```python
from build123d import *

# Parameters (mm, degrees)
BOSS_EXTRUDE1_DEPTH            = 101.6
CUT_EXTRUDE2_REACH             = 142.769
SKETCH2_R                      = 2.9845
CUT_EXTRUDE2_DIRECTION_2_DEPTH = 141.768746531
SKETCH8_W                      = 3.81
SKETCH8_H                      = 101.6
BOSS_EXTRUDE3_DEPTH            = 101.6
CUT_EXTRUDE5_DEPTH             = 4.572
SKETCH24_W                     = 38.1
SKETCH24_H                     = 35.56
BOSS_EXTRUDE8_DEPTH            = 7.62
BOSS_EXTRUDE8_TAPER            = 20
SKETCH29_W                     = 5.08
SKETCH29_H                     = 16.309015266
BOSS_EXTRUDE10_DEPTH           = 21.59
CUT_EXTRUDE8_DEPTH             = 199.322792527
CUT_EXTRUDE8_DEPTH_BACK        = 199.322792527
SKETCH30_R                     = 2.54
FILLET8_R                      = 2.38
CUT_EXTRUDE9_DEPTH             = 3.81
FILLET9_R                      = 2.54


with BuildPart() as part:
    # Sketch1 → Boss-Extrude1 (new body)
    with BuildSketch(Plane.XY):
        Polygon((0, 0), (0, 76.2), (60.71935441, 76.2), (60.71935441, 69.85), (6.35, 69.85), (6.35, 8.89), (60.71935441, 8.89), (60.71935441, 0), align=None)
    extrude(amount=BOSS_EXTRUDE1_DEPTH)

    # Sketch2 → Cut-Extrude2 (cut, up to next)
    with BuildSketch(Plane(origin=(0, 0, 0), x_dir=(1, 0, 0), z_dir=(0, 1, 0)), mode=Mode.PRIVATE) as cut_extrude2_sk1:
        with Locations(Location((30.359677205, -50.8, 0), (0, 0, 270))):
            Circle(SKETCH2_R)
    cut_extrude2_tool1 = extrude(cut_extrude2_sk1.sketch, amount=CUT_EXTRUDE2_REACH, mode=Mode.PRIVATE) & part.part
    add(cut_extrude2_tool1.solids().sort_by_distance((30.359677, 0, 50.8))[0], mode=Mode.SUBTRACT)

    # Sketch2 → Cut-Extrude2 direction 2 (cut)
    with BuildSketch(Plane(origin=(0, 0, 0), x_dir=(1, 0, 0), z_dir=(0, 1, 0))):
        with Locations(Location((30.359677205, -50.8, 0), (0, 0, 270))):
            Circle(SKETCH2_R)
    extrude(amount=-CUT_EXTRUDE2_DIRECTION_2_DEPTH, mode=Mode.SUBTRACT)

    # Sketch8 → Boss-Extrude3 (add)
    with BuildSketch(Plane(origin=(0, 76.2, 0), x_dir=(1, 0, 0), z_dir=(0, 1, 0))):
        with Locations((1.905, -50.8)):
            Rectangle(SKETCH8_W, SKETCH8_H)
    extrude(amount=BOSS_EXTRUDE3_DEPTH)

    # Sketch20 → Cut-Extrude5 (cut)
    with BuildSketch(Plane(origin=(0, 8.89, 0), x_dir=(1, 0, 0), z_dir=(0, 1, 0))):
        Polygon((35.462369538, -53.693279158), (35.416676623, -47.827578391), (30.31398429, -44.934299233), (25.256984872, -47.906720842), (25.302677788, -53.772421609), (30.405370121, -56.665700767), align=None)
    extrude(amount=-CUT_EXTRUDE5_DEPTH, mode=Mode.SUBTRACT)

    # Sketch24 → Boss-Extrude8 (add)
    with BuildSketch(Plane(origin=(3.81, 0, 0), x_dir=(0, 0, -1), z_dir=(1, 0, 0))):
        with Locations((-50.8, 160.02)):
            Rectangle(SKETCH24_W, SKETCH24_H)
    extrude(amount=BOSS_EXTRUDE8_DEPTH, taper=BOSS_EXTRUDE8_TAPER)

    # Sketch29 → Boss-Extrude10 (add)
    with BuildSketch(Plane(origin=(11.43, 0, 0), x_dir=(0, 0, -1), z_dir=(1, 0, 0))):
        with Locations((-60.96, 160.02)):
            Rectangle(SKETCH29_W, SKETCH29_H)
        with Locations((-50.8, 160.02)):
            Rectangle(SKETCH29_W, SKETCH29_H)
        with Locations((-40.64, 160.02)):
            Rectangle(SKETCH29_W, SKETCH29_H)
    extrude(amount=BOSS_EXTRUDE10_DEPTH)

    # Sketch30 → Cut-Extrude8 (cut, two sides: drawn at the far end of the back side and taken through both)
    with BuildSketch(Plane.XY.offset(63.5).offset(-CUT_EXTRUDE8_DEPTH_BACK)):
        with Locations(Location((22.225, 163.094507633, 0), (0, 0, 180))):
            Circle(SKETCH30_R)
    extrude(amount=CUT_EXTRUDE8_DEPTH + CUT_EXTRUDE8_DEPTH_BACK, mode=Mode.SUBTRACT)

    # Fillet8
    fillet8_edges = [part.edges().sort_by_distance(p)[0] for p in [
        (33.02, 168.174507633, 40.64),
        (11.43, 160.02, 43.18),
        (11.43, 151.865492367, 40.64),
        (33.02, 151.865492367, 40.64),
        (11.43, 168.174507633, 40.64),
        (11.43, 160.02, 38.1),
        (33.02, 168.174507633, 50.8),
        (11.43, 160.02, 53.34),
        (11.43, 151.865492367, 50.8),
        (33.02, 151.865492367, 50.8),
        (11.43, 168.174507633, 50.8),
        (11.43, 160.02, 48.26),
        (33.02, 168.174507633, 60.96),
        (11.43, 160.02, 63.5),
        (11.43, 151.865492367, 60.96),
        (33.02, 151.865492367, 60.96),
        (11.43, 168.174507633, 60.96),
        (11.43, 160.02, 58.42),
    ]]
    fillet(fillet8_edges, radius=FILLET8_R)

    # Sketch31 → Cut-Extrude9 (cut)
    with BuildSketch(Plane.XY.offset(63.5)):
        Polygon((26.416, 165.514182611), (22.225, 167.93385759), (18.034, 165.514182611), (18.034, 160.674832655), (22.225, 158.255157677), (26.416, 160.674832655), align=None)
    extrude(amount=-CUT_EXTRUDE9_DEPTH, mode=Mode.SUBTRACT)

    # Fillet9
    fillet9_edges = [part.edges().sort_by_distance(p)[0] for p in [
        (60.71935441, 4.445, 0),
        (6.35, 69.85, 50.8),
        (6.35, 8.89, 50.8),
        (60.71935441, 73.025, 101.6),
        (3.81, 76.2, 50.8),
        (1.905, 177.8, 101.6),
        (1.905, 177.8, 0),
        (60.71935441, 4.445, 101.6),
        (60.71935441, 73.025, 0),
    ]]
    fillet(fillet9_edges, radius=FILLET9_R)


solid = part.part
```
Can you work these out from the model? Positions are in its coordinate system, mm. A direction names the side the tool comes from. Coordinates: 2 decimals unless noted, no trailing zeros. Write each loop counter-clockwise with the first axis right and the second up, starting at its lowest first coordinate (ties: lowest second). Pieces come first, ordered by that corner, then holes. Notation, with made-up numbers: M 32.5,-11 L 41.5,-11 A19 cw 41.5,14 Z; hole C 70.25,-21.75 d5. An arc over 180 degrees is marked long. Answer as CSV lines item,"result".
Item 1: Please list where these lines run through material, in increasing order: line 1 along Z through (x, y) = (19, 158); line 2 along Y through (x, z) = (34.5, 26); line 3 along Y through (x, z) = (22, 60.5).
Geometry results:
line 1,"z = 38.1 to 43.18, 48.26 to 53.34, 58.42 to 63.5"
line 2,"y = 0 to 8.89, 69.85 to 76.2"
line 3,"y = 0 to 8.89, 69.85 to 76.2, 151.87 to 158.39, 167.8 to 168.17"
Item 2: We'd pull the mould along Y, two halves only. Please class faces 1 (the flat face through (60.719, 73, 50)), 2 (the flat face through (24.35, 166.707, 61.622)), 3 (the flat face through (38, 0, 50)), 4 (the flat face through (22, 168.175, 41)): +Y half, -Y half, draft (parallel to the pull), parting line (faces both ways), or undercut.
Geometry results:
face 1,"draft"
face 2,"undercut"
face 3,"-Y half"
face 4,"+Y half"
Item 3: Imagine slicing it at C-C on y = 98.5. List the corners of the cut face in (x, z) for me, plus the area to 3 significant figures.
Geometry results:
outline,"M 0,0 L 3.81,0 L 3.81,101.6 L 0,101.6 Z"
area,"387 mm2"
Item 4: On a 3-axis mill with a long thin cutter (end or side, diameter ignored), from which of +Z, -Z, +X, -X, +Y, -Y can I reach the whole of each face in a straight line? I mean faces 5 (the flat face through (33, 76.2, 50)), 6 (the flat face through (32.9, 6.6, 46.4)), 7 (the flat face through (33.02, 160, 51)), 8 (the flat face through (20.1, 159.48, 61.62)). Say none if no direction works.
Geometry results:
face 5,"+Z, -Z, +X"
face 6,"none"
face 7,"+Z, -Z, +X, +Y"
face 8,"+Z"
Item 5: Imagine slicing it at D-D on y = 62. List the corners of the cut face in (x, z) for me, plus the area to 3 significant figures.
Geometry results:
outline,"M 0,0 L 6.35,0 L 6.35,101.6 L 0,101.6 Z"
area,"645 mm2"
Item 6: I'm going to push flat-ended pins straight in: P1, Ø8, axis at x = 19.5, y = 158.5, coming from the -Z side; P2, Ø2.5, axis at x = 26.5, z = 62, coming from the +Y side; P3, Ø15.5, axis at x = 43, z = 67, coming from the -Y side; P4, Ø8, axis at x = 24.5, y = 164, coming from the +Z side. Where does each tip first touch, or does it pass through?
Geometry results:
P1,"stops at z = 38.1"
P2,"stops at y = 168.17"
P3,"stops at y = 0"
P4,"stops at z = 63.5"
Item 7: Imagine slicing it at A-A on x = 38. List the corners of the cut face in (y, z) for me, plus the area to 3 significant figures.
Geometry results:
outline,"M 0,0 L 8.89,0 L 8.89,101.6 L 0,101.6 Z; M 69.85,0 L 76.2,0 L 76.2,101.6 L 69.85,101.6 Z"
area,"1,550 mm2"
Item 8: Imagine slicing it at B-B on z = 50.8. State how many separate pieces and enclosed holes the cut face has, plus the area to 3 significant figures.
Geometry results:
separate pieces,"2"
enclosed holes,"1"
area,"2,210 mm2"
